```python
from build123d import *

# Parameters (mm, degrees)
F1_DEPTH    = 25.4
F2_SIZE     = 1.27
F3_T1_DEPTH = 62.588590634
F3_T3_DEPTH = 46.2433618017
F3_T5_DEPTH = 74.1232333831


# Not quite as in the source:
# - a fillet or chamfer that OpenCascade refuses, or shapes differently, is made with other operations: its cross-section is extruded or revolved along the edge and cut away or added


with BuildPart() as f1:
    # F0 (on Front) → F1 (new body)
    with BuildSketch(Plane.XZ):
        Polygon((0, 51.5181273222), (-48.1757372618, 33.8250361383), (-25.1621361822, 33.8250361383), (-25.1621361822, 0), align=None)
    extrude(amount=F1_DEPTH)

    # F2
    f2_edges = [f1.edges().sort_by_distance(p)[0] for p in [
        (-25.162136, -25.4, 16.912518),
        (-12.581068, -25.4, 25.759064),
        (-36.668937, -25.4, 33.825036),
        (-24.087869, -25.4, 42.671582),
    ]]
    chamfer(f2_edges, length=F2_SIZE)

    # F3: fillet of radius 1.778 on 3 edges, made by hand

    # F3_s2 → F3_t1 (cut)
    with BuildSketch(Plane.XZ.offset(-19.229295317)):
        with BuildLine():
            ThreePointArc((-21.78650907, 6.911415871), (-23.7845753127, 5.9593981498), (-25.1621361822, 7.6917181268))
            Line((-25.1621361822, 7.6917181268), (-25.1621361822, 0))
            Line((-25.1621361822, 0), (-21.78650907, 6.911415871))
        make_face()
    extrude(amount=F3_T1_DEPTH, mode=Mode.SUBTRACT)

    # F3_s4 → F3_t3 (cut)
    with BuildSketch(Plane.XZ.offset(-11.0566809008)):
        with BuildLine():
            ThreePointArc((-4.1515436611, 49.9934253721), (-2.2186732944, 49.5156925609), (-1.9409568164, 47.5441221078))
            Line((-1.9409568164, 47.5441221078), (0, 51.5181273222))
            Line((0, 51.5181273222), (-4.1515436611, 49.9934253721))
        make_face()
    extrude(amount=F3_T3_DEPTH, mode=Mode.SUBTRACT)

    # F3_s6 → F3_t5 (cut)
    with BuildSketch(Plane.XZ.offset(-24.9966166916)):
        with BuildLine():
            ThreePointArc((-38.7900503177, 37.2720371468), (-39.9276287585, 35.2917483238), (-38.1770905851, 33.8250361383))
            Line((-38.1770905851, 33.8250361383), (-48.1757372618, 33.8250361383))
            Line((-48.1757372618, 33.8250361383), (-38.7900503177, 37.2720371468))
        make_face()
    extrude(amount=F3_T5_DEPTH, mode=Mode.SUBTRACT)


solid = f1.part
```
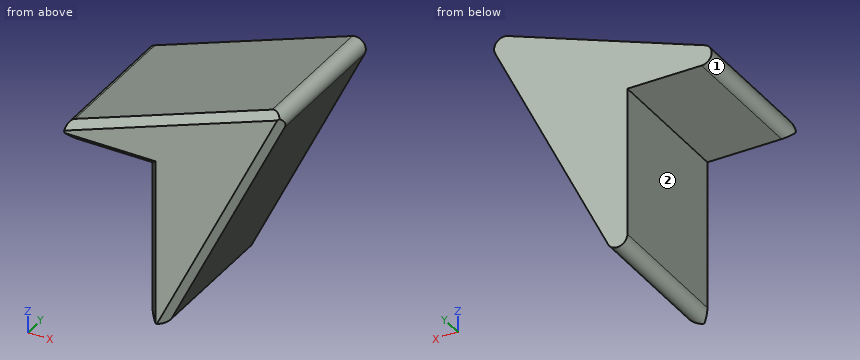
Verification items for the finished model (mm, model axes). Face numbers are marked on the shaded views. A direction names the side the tool comes from. Give positions to 0.01 mm unless a question says otherwise; leave off trailing zeros. Order: outer loops, then holes, each group sorted by start corner. A loop starts at its lowest first (then second) coordinate and runs counter-clockwise, first axis right, second up. Notation, with made-up numbers: M 14,41.5 L 31,41.5 A10 ccw 31,48.5 Z; hole C 29,53 d5. An arc over 180 degrees is marked long. Answer in a Markdown table with one row per item. Add a question column.
Item 1: Section check A-A, the plane y = -4.5. Enter the section's corners in (x, z), and give its area (3 significant figures).
Item 2: Scan lines: probe 1 along Z at (x, y) = (-32, -2.75); probe 2 along X at (y, z) = (-16.5, 26.5); probe 3 along Z at (x, y) = (-8, -15). Record each from-to range of solid material in increasing order. Write a range as from..to.
Item 3: Tool access check on the marked faces 1 and 2. Record the directions out of +Z, -Z, +X, -X, +Y, -Y that give a thin tool (end or side, any length) a straight path to the whole face; none if there is none.
Item 4: Section check B-B, the plane x = -33.5. Enter the section's corners in (y, z).
Item 5: Gauge pin test, flat ends, axial feed: pin 1 (1.5 mm diameter, centred on x = -33, y = -15, fed in from -Z); pin 2 (14.5 mm diameter, centred on x = -32, y = -17.5, fed in from -Z); pin 3 (5 mm diameter, centred on x = -9.5, y = -9, fed in from +Z). Record the tip position at first contact, or that the pin passes through.
Item 6: Section check C-C, the plane z = 36.5. Enter the section's corners in (x, y).
Filled sheet:
| question | item | result |
|---|---|---|
| 1 | outline | M -38.79,37.27 A1.78 ccw -38.18,33.83 L -25.16,33.83 L -25.16,7.69 A1.78 ccw -21.79,6.91 L -1.94,47.54 A1.78 ccw -4.15,49.99 Z |
| 1 | area | 602 mm^2 |
| 2 | probe 1 | z = 33.83..39.77 |
| 2 | probe 2 | x = -25.16..-12.22 |
| 2 | probe 3 | z = 35.14..48.58 |
| 3 | face 1 | -X, +Y, -Y |
| 3 | face 2 | -Z, -X, +Y, -Y |
| 4 | outline | M -25.4,35.1 L -24.13,33.83 L 0,33.83 L 0,39.21 L -24.13,39.21 L -25.4,37.86 Z |
| 5 | pin 1 | stops at z = 33.83 |
| 5 | pin 2 | stops at z = 6.55 |
| 5 | pin 3 | stops at z = 48.95 |
| 6 | outline | M -39.71,-24.54 L -37.21,-25.4 L -8.75,-25.4 L -7.34,-24.13 L -7.34,0 L -39.71,0 Z |
